from build123d import *

# Parameters (mm, degrees)
MAIN_BODY_SKETCH_R     = 117.99951
MAIN_BODY_DEPTH        = 3.175
TABS_SKETCH_W          = 6.35
TABS_SKETCH_H          = 152.4
TABS_SKETCH_W_2        = 152.4
TABS_SKETCH_H_2        = 6.35
OUTSIDE_TABS_DEPTH     = 6.35
F_6_0_204_TUBE_MOUNT_D = 5.1816
SKETCH12_W             = 165.1
SKETCH12_H             = 50.8
BOSS_EXTRUDE1_DEPTH    = 6.35
SKETCH13_R             = 1.5
CUT_EXTRUDE1_DEPTH     = 489.042014073
SKETCH14_W             = 6.35
SKETCH14_H             = 12.7
CUT_EXTRUDE2_DEPTH     = 489.042014073
SKETCH15_W             = 87.70313901
SKETCH15_H             = 6.35
CUT_EXTRUDE3_DEPTH     = 489.042014073
SKETCH16_R             = 1.8
SKETCH16_R_2           = 2.159
SKETCH16_W             = 10
SKETCH16_H             = 6
CUT_EXTRUDE4_DEPTH     = 489.042014073
SKETCH18_W             = 158.75
SKETCH18_H             = 10.820932089
CUT_EXTRUDE6_DEPTH     = 489.042014073
FILLET1_R              = 25.4


with BuildPart() as part:
    # Main Body Sketch → Main Body (new, symmetric)
    with BuildSketch(Plane.XY):
        with BuildLine():
            Line((-96.545932089, -95.25), (-254, -95.25))
            Line((-254, -95.25), (-254, 95.25))
            Line((-254, 95.25), (-96.545932089, 95.25))
            ThreePointArc((-96.545932089, 95.25), (0, 135.6233), (96.545932089, 95.25))
            Line((96.545932089, 95.25), (254, 95.25))
            Line((254, 95.25), (254, -95.25))
            Line((254, -95.25), (96.545932089, -95.25))
            ThreePointArc((96.545932089, -95.25), (95.900155117, -95.900155117), (95.25, -96.545932089))
            Line((95.25, -96.545932089), (95.25, -406.4))
            Line((95.25, -406.4), (-95.25, -406.4))
            Line((-95.25, -406.4), (-95.25, -96.545932089))
            ThreePointArc((-95.25, -96.545932089), (-95.900155117, -95.900155117), (-96.545932089, -95.25))
        make_face()
        Circle(MAIN_BODY_SKETCH_R, mode=Mode.SUBTRACT)
    extrude(amount=MAIN_BODY_DEPTH, both=True)

    # Tabs Sketch → Outside Tabs (add)
    with BuildSketch(Plane.XY.offset(3.175)):
        with Locations((-257.175, 0)):
            Rectangle(TABS_SKETCH_W, TABS_SKETCH_H)
        with Locations((0, -409.575)):
            Rectangle(TABS_SKETCH_W_2, TABS_SKETCH_H_2)
    outside_tabs = extrude(amount=-OUTSIDE_TABS_DEPTH)

    # Outside Tabs Mirror: Outside Tabs across plane
    add(outside_tabs.mirror(Plane(origin=(0, 0, 0), x_dir=(0, 0, 1), z_dir=(1, 0, 0))))

    # #6 (0.204) Tube Mount (through all)
    with Locations(Plane.XY.offset(3.175)):
        with Locations((0, -123.19), (123.19, 0), (0, 123.19), (-123.19, 0)):
            Hole(F_6_0_204_TUBE_MOUNT_D / 2)

    # Sketch12 → Boss-Extrude1 (add)
    with BuildSketch(Plane.XY.offset(3.175)):
        with Locations((-177.8, -342.9)):
            Rectangle(SKETCH12_W, SKETCH12_H)
        with Locations((177.8, -342.9)):
            Rectangle(SKETCH12_W, SKETCH12_H)
    extrude(amount=-BOSS_EXTRUDE1_DEPTH)

    # Sketch13 → Cut-Extrude1 (cut, through all)
    with BuildSketch(Plane.XY.offset(3.175)):
        with Locations((-196.85, -333.4)):
            Circle(SKETCH13_R)
        with Locations((-187.35, -342.9)):
            Circle(SKETCH13_R)
        with Locations((-196.85, -352.4)):
            Circle(SKETCH13_R)
        with Locations((-206.35, -342.9)):
            Circle(SKETCH13_R)
    cut_extrude1 = extrude(amount=-CUT_EXTRUDE1_DEPTH, mode=Mode.SUBTRACT)

    # Mirror2: Cut-Extrude1 across plane
    add(cut_extrude1.mirror(Plane(origin=(0, 0, 0), x_dir=(0, 0, 1), z_dir=(1, 0, 0))), mode=Mode.SUBTRACT)

    # Sketch14 → Cut-Extrude2 (cut, through all)
    with BuildSketch(Plane.XY.offset(3.175)):
        with Locations((-257.175, -323.85)):
            Rectangle(SKETCH14_W, SKETCH14_H)
        with Locations((-257.175, -361.95)):
            Rectangle(SKETCH14_W, SKETCH14_H)
    cut_extrude2 = extrude(amount=-CUT_EXTRUDE2_DEPTH, mode=Mode.SUBTRACT)

    # Mirror3: Cut-Extrude2 across plane
    add(cut_extrude2.mirror(Plane(origin=(0, 0, 0), x_dir=(0, 0, 1), z_dir=(1, 0, 0))), mode=Mode.SUBTRACT)

    # Sketch15 → Cut-Extrude3 (cut, through all)
    with BuildSketch(Plane.XY.offset(3.175)):
        with Locations((-133.948430495, -73.025)):
            Rectangle(SKETCH15_W, SKETCH15_H)
        with Locations((133.948430495, -73.025)):
            Rectangle(SKETCH15_W, SKETCH15_H)
    extrude(amount=-CUT_EXTRUDE3_DEPTH, mode=Mode.SUBTRACT)

    # Sketch16 → Cut-Extrude4 (cut, through all)
    with BuildSketch(Plane.XY.offset(3.175)):
        with Locations((-25.5, -152.39951)):
            Circle(SKETCH16_R)
        with Locations(Location((-25.5, -191.39951, 0), (0, 0, 180))):
            Circle(SKETCH16_R)
        with Locations((25.5, -191.39951)):
            Circle(SKETCH16_R)
        with Locations(Location((25.5, -152.39951, 0), (0, 0, 180))):
            Circle(SKETCH16_R)
        with Locations((-9.795, -213.74951)):
            Circle(SKETCH16_R_2)
        with Locations(Location((-9.795, -293.74951, 0), (0, 0, 180))):
            Circle(SKETCH16_R_2)
        with Locations(Location((9.795, -213.74951, 0), (0, 0, 180))):
            Circle(SKETCH16_R_2)
        with Locations((9.795, -293.74951)):
            Circle(SKETCH16_R_2)
        with Locations((-4, -182.89951)):
            Rectangle(SKETCH16_W, SKETCH16_H)
    extrude(amount=-CUT_EXTRUDE4_DEPTH, mode=Mode.SUBTRACT)

    # Sketch18 → Cut-Extrude6 (cut, through all)
    with BuildSketch(Plane.XY.offset(3.175)):
        with Locations((-174.625, -91.135466045)):
            Rectangle(SKETCH18_W, SKETCH18_H)
    cut_extrude6 = extrude(amount=-CUT_EXTRUDE6_DEPTH, mode=Mode.SUBTRACT)

    # Mirror4: Cut-Extrude6 across plane
    add(cut_extrude6.mirror(Plane(origin=(0, 0, 0), x_dir=(0, 0, 1), z_dir=(1, 0, 0))), mode=Mode.SUBTRACT)

    # Fillet1
    fillet1_edges = [part.edges().sort_by_distance(p)[0] for p in [
        (-95.25, -317.5, 0),
        (-95.25, -368.3, 0),
        (95.25, -317.5, 0),
        (95.25, -368.3, 0),
        (-96.545932089, 95.25, 0),
        (96.545932089, 95.25, 0),
        (-95.25, -85.725, 0),
        (95.25, -85.725, 0),
    ]]
    fillet(fillet1_edges, radius=FILLET1_R)


solid = part.part
Verification items for the finished model (mm, model axes). A direction names the side the tool comes from. Coordinates: 2 decimals unless noted, no trailing zeros. Order: outer loops, then holes, each group sorted by start corner. A loop starts at its lowest first (then second) coordinate and runs counter-clockwise, first axis right, second up. Notation, with made-up numbers: M 15.5,28 L 57.5,28 A24 ccw 57.5,67 Z; hole C -1,27 d7. An arc over 180 degrees is marked long. One line per item, written item: value. Start each with the question number.
Item 1: Sectioned sample at A-A (x = -151.5). Enter the section's corners in (y, z) (3 decimals).
Item 2: Sectioned sample at C-C (y = -230). Enter the section's corners in (x, z) (3 decimals).
Item 3: Sectioned sample at D-D (z = 1.75). Count the separate pieces of the cut face and the enclosed holes in it, then the cut area to 3 significant figures.
Item 4: Mould release check, pull along Y, two halves, no side actions. Record for faces 1 (the cylindrical face through (102.49, -375.94, -0.04)), 2 (the cylindrical face through (-102.49, -309.86, -0.04)), 3 (the flat face through (4, -135, -3.175)): released by +Y, released by -Y, zero draft, split by the parting line, or undercut.
Item 5: Gauge pin test, flat ends, axial feed: pin 1 (3 mm diameter, centred on y = 86, z = 1, fed in from -X); pin 2 (1.9 mm diameter, centred on x = -168, z = 0, fed in from -Y); pin 3 (2 mm diameter, centred on x = 25.5, y = -191.4, fed in from -Z); pin 4 (3 mm diameter, centred on x = -151, z = 1, fed in from +Y). Record the tip position at first contact, or that the pin passes through.
Item 6: Scan lines: probe 1 along Y at (x, z) = (-196.85, 1.25) (3 decimals); probe 2 along Y at (x, z) = (-187.35, 0) (3 decimals); probe 3 along Y at (x, z) = (-123.19, 0.25) (3 decimals). Record each from-to range of solid material in increasing order.
Item 7: Access from +Z, -Z, +X, -X, +Y, -Y to the whole of each face (thin tool, end or side, straight path). Record for faces 4 (the cylindrical face through (102.493, -93.363, -0.044)), 5 (the cylindrical face through (-102.888, -92.968, -0.044)), 6 (the cylindrical face through (-1.374, 135.616, 0.044)), 7 (the cylindrical face through (-1.44, -117.99, -0.04)).
Item 8: Sectioned sample at B-B (y = 37.5). Enter the section's corners in (x, z) (3 decimals), then the cut area to 3 significant figures.
Conclusion:
1. outline: M -368.3,-3.175 L -317.5,-3.175 L -317.5,3.175 L -368.3,3.175 Z; M -85.725,-3.175 L -76.2,-3.175 L -76.2,3.175 L -85.725,3.175 Z; M -69.85,-3.175 L 95.25,-3.175 L 95.25,3.175 L -69.85,3.175 Z
2. outline: M -95.25,-3.175 L 95.25,-3.175 L 95.25,3.175 L -95.25,3.175 Z
3. separate pieces: 1
3. enclosed holes: 22
3. area: 133,000 mm^2
4. face 1: released by -Y
4. face 2: undercut
4. face 3: zero draft
5. pin 1: stops at x = -254
5. pin 2: stops at y = -368.3
5. pin 3: passes through
5. pin 4: stops at y = 95.25
6. probe 1: y = -368.3 to -353.9, -350.9 to -334.9, -331.9 to -317.5, -85.725 to 95.25
6. probe 2: y = -368.3 to -344.4, -341.4 to -317.5, -85.725 to 95.25
6. probe 3: y = -368.3 to -317.5, -85.725 to -76.2, -69.85 to -2.591, 2.591 to 95.25
7. face 4: +Z, -Z, +X
7. face 5: +Z, -Z, -X
7. face 6: +Z, -Z, +Y
7. face 7: +Z, -Z
8. outline: M -260.35,-3.175 L -111.882,-3.175 L -111.882,3.175 L -260.35,3.175 Z; M 111.882,-3.175 L 260.35,-3.175 L 260.35,3.175 L 111.882,3.175 Z
8. area: 1,890 mm^2
